Model file for the job. Use its own axes, mm. A direction names the side the tool comes from. Round coordinates to 2 decimals unless told otherwise and drop trailing zeros. Order: outer loops, then holes, each group sorted by start corner. A loop starts at its lowest first (then second) coordinate and runs counter-clockwise, first axis right, second up. Notation, with made-up numbers: (-26.5, -35) -> (22.5, -35) arc R26 ccw to (22.5, -10) -> close; hole circle Ø4 at (-36.5, -35.5). An arc over 180 degrees is marked (long way). Answer as CSV lines item,"result".
```python
from build123d import *

# Parameters (mm, degrees)
RESSALTO_EXTRUS_O1_DEPTH                             = 1000
CORTE_EXTRUS_O1_START                                = -1000
CORTE_EXTRUS_O1_DEPTH                                = 1000
CORTE_EXTRUS_O2_DEPTH                                = 1001.031261626
CORTE_EXTRUS_O3_DEPTH                                = 1001.031261626
CORTE_EXTRUS_O4_DEPTH                                = 1001.031261626
CORTE_EXTRUS_O5_DEPTH                                = 0.002166667
CORTE_EXTRUS_O6_DEPTH                                = 0.002166667
CORTE_EXTRUS_O7_DEPTH                                = 0.002166667
CORTE_EXTRUS_O8_DEPTH                                = 0.002166667
INCLINA_O1_ANGLE                                     = 45.1469538
ESBO_O10_W                                           = 0.450000001
ESBO_O10_H                                           = 1000
REBAIXO_PARA_PARAFUSO_DE_M_QUINA_DE_CABE_D           = 3.5
REBAIXO_PARA_PARAFUSO_DE_M_QUINA_DE_CABE_CBORE_D     = 6
REBAIXO_PARA_PARAFUSO_DE_M_QUINA_DE_CABE_CBORE_DEPTH = 3.50000002
CHANFRO1_SIZE                                        = 0.062563219
CHANFRO1_SIZE2                                       = 0.062205617
CHANFRO3_START                                       = -3.730761794
CHANFRO3_DEPTH                                       = 0.399013115
CHANFRO4_SIZE                                        = 0.4
FILETE1_R                                            = 0.130000023
SKETCH1_W                                            = 36.072768502
SKETCH1_H                                            = 771.589023544
SKETCH1_W_2                                          = 21.632087489
SKETCH1_H_2                                          = 231.614654652
CUT_EXTRUDE1_DEPTH                                   = 10


with BuildPart() as part:
    # Esboço1 → Ressalto-extrusão1 (new body)
    with BuildSketch(Plane.XZ):
        with BuildLine():
            Line((4.5, 5.4097155), (4.5, 6.01167813))
            Line((4.5, 6.01167813), (4.1, 6.50000002))
            Line((4.1, 6.50000002), (-4.1, 6.50000002))
            Line((-4.1, 6.50000002), (-4.5, 6.01167813))
            Line((-4.5, 6.01167813), (-4.5, 2e-08))
            Line((-4.5, 2e-08), (4.5, 2e-08))
            Line((4.5, 2e-08), (4.5, 3.50196265))
            ThreePointArc((4.5, 3.50196265), (4.477413879, 3.553810372), (4.43494978, 3.59116167))
            ThreePointArc((4.43494978, 3.59116167), (3.930462682, 4.43021964), (4.43494978, 5.26927761))
            ThreePointArc((4.43494978, 5.26927761), (4.490651601, 5.328761203), (4.5, 5.4097155))
        make_face()
    extrude(amount=-RESSALTO_EXTRUS_O1_DEPTH)

    # Esboço2 → Corte-extrusão1 (cut)
    with BuildSketch(Plane(origin=(0, 1000, 0), x_dir=(-1, 0, 0), z_dir=(0, 1, 0)).offset(CORTE_EXTRUS_O1_START)):
        with BuildLine():
            Line((-4.030498711, 4.00588336), (-3.673447948, 4.00588336))
            ThreePointArc((-3.673447948, 4.00588336), (-3.223447946, 4.455883362), (-3.673447948, 4.905883363))
            Line((-3.673447948, 4.905883363), (-3.953580008, 4.905883363))
            ThreePointArc((-3.953580008, 4.905883363), (-4.010719931, 4.899199784), (-4.065149208, 4.917830263))
            ThreePointArc((-4.065149208, 4.917830263), (-3.93114763, 4.466290066), (-4.030498711, 4.00588336))
        make_face()
    extrude(amount=CORTE_EXTRUS_O1_DEPTH, mode=Mode.SUBTRACT)

    # Esboço3 → Corte-extrusão2 (cut, through all)
    with BuildSketch(Plane(origin=(0, 1000, 0), x_dir=(-1, 0, 0), z_dir=(0, 1, 0))):
        with BuildLine():
            Line((4.5, 4.03150278), (4.5, 4.88017535))
            Line((4.5, 4.88017535), (3.66946318, 4.88017535))
            ThreePointArc((3.66946318, 4.88017535), (3.969667593, 4.455839065), (3.66946318, 4.03150278))
            Line((3.66946318, 4.03150278), (4.5, 4.03150278))
        make_face()
    extrude(amount=-CORTE_EXTRUS_O2_DEPTH, mode=Mode.SUBTRACT)

    # Esboço4 → Corte-extrusão3 (cut, through all)
    with BuildSketch(Plane(origin=(0, 1000, 0), x_dir=(-1, 0, 0), z_dir=(0, 1, 0))):
        with BuildLine():
            Line((4.026513974, 4.88017535), (4.5, 4.88017535))
            Line((4.5, 4.88017535), (4.5, 5.328056964))
            ThreePointArc((4.5, 5.328056964), (4.223646078, 5.145991535), (4.026513974, 4.88017535))
        make_face()
    extrude(amount=-CORTE_EXTRUS_O3_DEPTH, mode=Mode.SUBTRACT)

    # Esboço5 → Corte-extrusão4 (cut, through all)
    with BuildSketch(Plane(origin=(0, 1000, 0), x_dir=(-1, 0, 0), z_dir=(0, 1, 0))):
        with BuildLine():
            Line((4.5, 3.583620931), (4.5, 4.03150278))
            Line((4.5, 4.03150278), (4.026513856, 4.03150278))
            ThreePointArc((4.026513856, 4.03150278), (4.223645982, 3.76568645), (4.5, 3.583620931))
        make_face()
    extrude(amount=-CORTE_EXTRUS_O4_DEPTH, mode=Mode.SUBTRACT)

    # Esboço6 → Corte-extrusão5 (cut)
    with BuildSketch(Plane(origin=(0, 1000, 0), x_dir=(-1, 0, 0), z_dir=(0, 1, 0))):
        Polygon((0.891369267, 3.403698133), (0.714701433, 3.168235633), (0.2187042, 2.61105), (1.0945792, 2.61105), (1.0945792, 2.695983333), (0.398689633, 2.695983333), (0.794326433, 3.149466667), (0.9743123, 3.3891), (1.067110588, 3.573407857), (0.95413722, 3.802321701), (0.7876908, 3.88505), (0.54301, 3.88505), (0.375434678, 3.803592619), (0.295011167, 3.6384023), (0.295011167, 3.562), (0.3812718, 3.562), (0.3812718, 3.631766667), (0.437672733, 3.743620833), (0.549645633, 3.800116667), (0.7802262, 3.800116667), (0.893028067, 3.743810633), (0.976240026, 3.576039029), align=None)
    extrude(amount=-CORTE_EXTRUS_O5_DEPTH, mode=Mode.SUBTRACT)

    # Esboço7 → Corte-extrusão6 (cut)
    with BuildSketch(Plane.XZ):
        Polygon((-0.214632167, 3.88505), (-0.953983333, 3.88505), (-0.953983333, 2.61105), (-0.214632167, 2.61105), (-0.214632167, 2.695983333), (-0.86905, 2.695983333), (-0.86905, 3.205583333), (-0.5123963, 3.205583333), (-0.5123963, 3.290516667), (-0.86905, 3.290516667), (-0.86905, 3.800116667), (-0.214632167, 3.800116667), align=None)
    extrude(amount=-CORTE_EXTRUS_O6_DEPTH, mode=Mode.SUBTRACT)

    # Esboço8 → Corte-extrusão7 (cut)
    with BuildSketch(Plane(origin=(0, 1000, 0), x_dir=(-1, 0, 0), z_dir=(0, 1, 0))):
        Polygon((-0.214632167, 3.88505), (-0.953983333, 3.88505), (-0.953983333, 2.61105), (-0.214632167, 2.61105), (-0.214632167, 2.695983333), (-0.86905, 2.695983333), (-0.86905, 3.205583333), (-0.5123963, 3.205583333), (-0.5123963, 3.290516667), (-0.86905, 3.290516667), (-0.86905, 3.800116667), (-0.214632167, 3.800116667), align=None)
    extrude(amount=-CORTE_EXTRUS_O7_DEPTH, mode=Mode.SUBTRACT)

    # Esboço9 → Corte-extrusão8 (cut)
    with BuildSketch(Plane.XZ):
        Polygon((0.510057167, 3.620830633), (0.6071, 3.718655633), (0.6071, 2.609403333), (0.692033333, 2.609403333), (0.692033333, 3.883403333), (0.6741176, 3.883403333), (0.6741176, 3.795069794), (0.3690544, 3.640736667), (0.3690544, 3.551253333), align=None)
    extrude(amount=-CORTE_EXTRUS_O8_DEPTH, mode=Mode.SUBTRACT)

    # Inclinação1
    inclina_o1_faces = [part.faces().sort_by_distance(p)[0] for p in [
        (0.6741176, 0.001083333, 3.839236564),
    ]]
    draft(inclina_o1_faces, Plane(origin=(0.692033333, 0.002166667, 3.883403333), x_dir=(-1, 0, 0), z_dir=(0, 0, -1)), INCLINA_O1_ANGLE)

    # Esboço10 → Corte-Revolução1 (revolve, cut)
    with BuildSketch(Plane.XY.offset(4.455839065)):
        with Locations((-3.294667591, 500)):
            Rectangle(ESBO_O10_W, ESBO_O10_H)
    revolve(axis=Axis((-3.519667591, 1000, 4.455839065), (0, -1, 0)), mode=Mode.SUBTRACT)

    # Rebaixo para parafuso de máquina de cabeça sextavada de M31 (through all)
    with Locations(Plane.XY.offset(6.50000002)):
        with Locations((0, 221.298822188), (0, 201.298822188), (0, 241.298822188), (0, 261.298822188)):
            CounterBoreHole(REBAIXO_PARA_PARAFUSO_DE_M_QUINA_DE_CABE_D / 2, REBAIXO_PARA_PARAFUSO_DE_M_QUINA_DE_CABE_CBORE_D / 2, REBAIXO_PARA_PARAFUSO_DE_M_QUINA_DE_CABE_CBORE_DEPTH)

    # Chanfro1
    chanfro1_edges = [part.edges().sort_by_distance(p)[0] for p in [
        (-0.976240026, 999.998916667, 3.576039029),
    ]]
    chanfro1_side = [part.faces().sort_by_distance(p)[0] for p in [
        (-0.933804646, 999.998916667, 3.489868581),
    ]]
    chamfer(chanfro1_edges, length=CHANFRO1_SIZE, length2=CHANFRO1_SIZE2, reference=chanfro1_side[0])

    # Chanfro3: read off the stored shape, not the designer's step
    # Chanfro3 outline → Chanfro3 (add)
    with BuildSketch(Plane(origin=(0, 0, 0), x_dir=(0.8991051825477068, 0, 0.43773264753254887), z_dir=(0.4377326475325489, 0, -0.8991051825477069)).offset(CHANFRO3_START)):
        Polygon((1.327401403, -999.997833333), (1.31122788, -999.997833333), (1.311999664, -1000), (1.327401403, -1000), align=None)
    extrude(amount=CHANFRO3_DEPTH)

    # Chanfro4
    chanfro4_edges = [part.edges().sort_by_distance(p)[0] for p in [
        (4.5, 500, 2e-08),
        (-4.5, 500, 2e-08),
    ]]
    chamfer(chanfro4_edges, length=CHANFRO4_SIZE)

    # Filete1
    filete1_edges = [part.edges().sort_by_distance(p)[0] for p in [
        (4.030498711, 500, 4.00588336),
        (-4.026513974, 500, 4.88017535),
        (-4.5, 500, 5.328056964),
        (-4.5, 500, 3.583620931),
        (-4.026513856, 500, 4.03150278),
    ]]
    fillet(filete1_edges, radius=FILETE1_R)

    # Sketch1 → Cut-Extrude1 (cut)
    with BuildSketch(Plane(origin=(0, 0, 0), x_dir=(-1, 0, 0), z_dir=(0, 0, -1))):
        with Locations((-9.39117436, 624.361983818)):
            Rectangle(SKETCH1_W, SKETCH1_H)
        with Locations((0.25600221, 82.81425767)):
            Rectangle(SKETCH1_W_2, SKETCH1_H_2)
    extrude(amount=-CUT_EXTRUDE1_DEPTH, mode=Mode.SUBTRACT)


solid = part.part
```
Q1. Wall check: L1, parallel to Y at x = 0, z = 1.6; L2, parallel to Y at x = 0, z = 4.2; L3, parallel to Z at x = 3.5, y = 209. Give the ranges that are in metal, low to high. Write a range as [from, to].
Checks:
L1,"[198.62, 199.55], [203.05, 219.55], [223.05, 238.57]"
L2,"[204.3, 218.3], [224.3, 238.3]"
L3,"[0, 4.04], [4.87, 6.5]"
Q2. Flat gauge pins, fed straight in: pin 1 (1.6 mm diameter, centred on y = 216.5, z = 2.5, fed in from +X); pin 2 (3 mm diameter, centred on x = 0, y = 220, fed in from +Z). Where does each tip first touch, or does it go through?
Checks:
pin 1,"x = 4.5"
pin 2,"z = 3"
Q3. Saw through at B-B (y = 206). Write the cut outline in (x, z).
Checks:
outline,"(-4.5, 0.4) -> (-4.1, 0) -> (4.1, 0) -> (4.5, 0.4) -> (4.5, 3.5) arc R0.13 ccw to (4.43, 3.59) arc R0.95 cw to (4.07, 3.94) arc R0.13 ccw to (3.95, 4.01) -> (3.67, 4.01) arc R0.45 cw to (3.67, 4.91) -> (3.95, 4.91) arc R0.13 ccw to (4.07, 4.92) arc R0.95 cw to (4.43, 5.27) arc R0.13 ccw to (4.5, 5.41) -> (4.5, 6.01) -> (4.1, 6.5) -> (-4.1, 6.5) -> (-4.5, 6.01) -> (-4.5, 5.41) arc R0.13 ccw to (-4.43, 5.29) arc R0.95 cw to (-4.06, 4.94) arc R0.13 ccw to (-3.95, 4.88) -> (-3.67, 4.88) arc R0.45 cw (long way) to (-3.67, 4.03) -> (-3.95, 4.03) arc R0.13 ccw to (-4.06, 3.97) arc R0.95 cw to (-4.43, 3.62) arc R0.13 ccw to (-4.5, 3.5) -> close"
Q4. Tool access for faces 1 (the flat face through (4.5, 218, 2)), 2 (the cylindrical face through (-0.391, 224.273, 4.775)), 3 (the cylindrical face through (0, 238.3, 4.8)): list every direction of +Z, -Z, +X, -X, +Y, -Y with a clear straight run to the whole face (end or side of a thin tool).
Checks:
face 1,"+Z, -Z, +X, +Y, -Y"
face 2,"+Z"
face 3,"+Z, +Y"
Q5. Saw through at A-A (x = 0). Write the cut outline in (y, z), plus the area to 3 significant figures.
Checks:
outline,"(198.62, 0) -> (199.55, 0) -> (199.55, 3) -> (198.62, 3) -> close; (203.05, 0) -> (219.55, 0) -> (219.55, 3) -> (218.3, 3) -> (218.3, 6.5) -> (204.3, 6.5) -> (204.3, 3) -> (203.05, 3) -> close; (223.05, 0) -> (238.57, 0) -> (238.57, 3) -> (238.3, 3) -> (238.3, 6.5) -> (224.3, 6.5) -> (224.3, 3) -> (223.05, 3) -> close"
area,"197 mm²"
Q6. Mould opens along X. For faces 4 (the flat face through (0, 238.567, 2)), 5 (the cylindrical face through (3.224, 218.315, 4.446)), 6 (the flat face through (0, 219, 3)) say: +X half, -X half, draft (parallel to the pull), parting line (faces both ways), or undercut.
Checks:
face 4,"draft"
face 5,"+X half"
face 6,"undercut"
